Verification items for this drawing (mm, ordinates from the low corner). A direction names the side the tool comes from. Coordinates: 2 decimals unless noted, no trailing zeros. Order: outer loops, then holes, each group sorted by start corner. A loop starts at its lowest first (then second) coordinate and runs counter-clockwise, first axis right, second up. Notation, with made-up numbers: (74, 47) - (85, 47) arc R17 ccw to (85, 79) - close; hole circle Ø7 at (-17, 50). An arc over 180 degrees is marked (long way). Use CSV: the item, a comma, the result in double quotes. Start each with the question number.
1) Sectioned sample at C-C, the plane x = 14. Record the cut outline in (y, z), and give its area (3 significant figures).
2) Sectioned sample at B-B, the plane y = 5.5. Record the cut outline in (x, z).
3) Sectioned sample at A-A, the plane z = 2.25. Record the cut outline in (x, y).
4) Thickness scan on probe 1 along X at (y, z) = (5.5, 4.75); probe 2 along X at (y, z) = (7, 5.5); probe 3 along X at (y, z) = (3.25, 2.25). Record the ranges inside material, lowest first. Write a range as [from, to].
5) Tool access check on the marked faces 4, 5, 6, 7 and 8. Record the directions out of +Z, -Z, +X, -X, +Y, -Y that give a thin tool (end or side, any length) a straight path to the whole face; none if there is none.
6) Draft check along X on the marked faces 1, 2 and 3. Enter one of: released by +X, released by -X, zero draft, split by the parting line, or undercut.
7) Sectioned sample at D-D, the plane y = 10.75. Record the cut outline in (x, z), and give its area (3 significant figures).
8) Depth check by flat-ended pin: P1, Ø1.5, axis at y = 7.5, z = 3.5, coming from the -X side; P2, Ø4, axis at x = 17.5, y = 2, coming from the +Z side; P3, Ø2, axis at x = 31.5, y = 12, coming from the +Z side; P4, Ø1.5, axis at x = 16.5, z = 5.5, coming from the +Y side. Enter the tip coordinate at first touch or a pass-through.
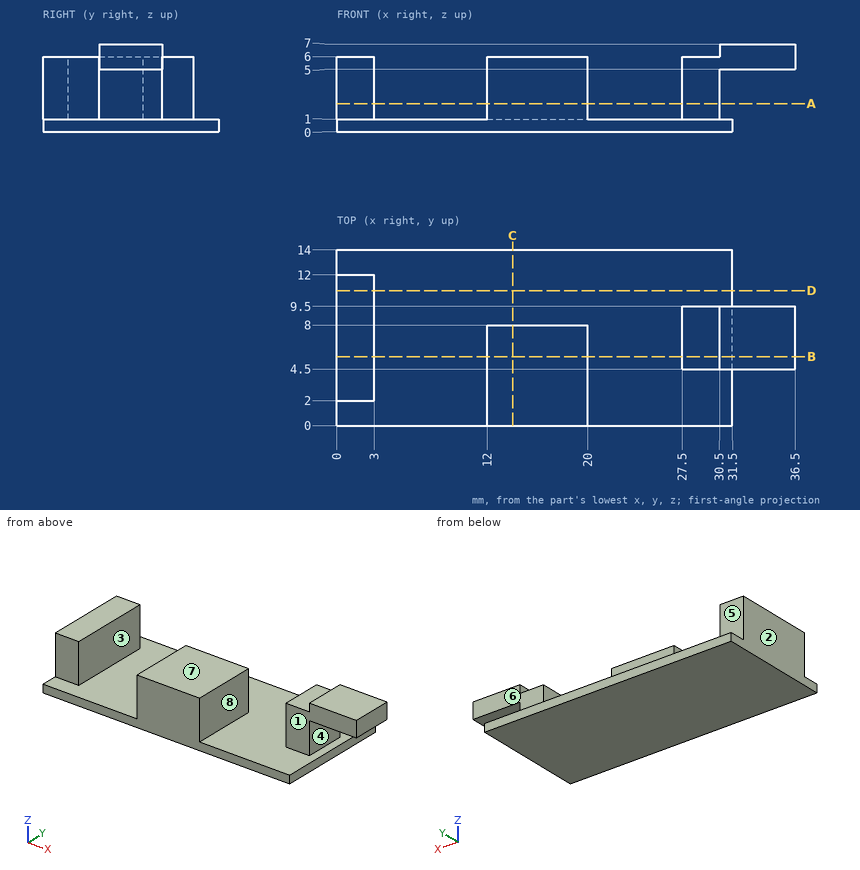
Evaluation:
1,outline,"(0, 0) - (14, 0) - (14, 1) - (8, 1) - (8, 6) - (0, 6) - close"
1,area,"54.0 mm²"
2,outline,"(0, 0) - (31.5, 0) - (31.5, 1) - (30.5, 1) - (30.5, 5) - (36.5, 5) - (36.5, 7) - (30.5, 7) - (30.5, 6) - (27.5, 6) - (27.5, 1) - (20, 1) - (20, 6) - (12, 6) - (12, 1) - (3, 1) - (3, 6) - (0, 6) - close"
3,outline,"(0, 2) - (3, 2) - (3, 12) - (0, 12) - close; (12, 0) - (20, 0) - (20, 8) - (12, 8) - close; (27.5, 4.5) - (30.5, 4.5) - (30.5, 9.5) - (27.5, 9.5) - close"
4,probe 1,"[0, 3], [12, 20], [27.5, 30.5]"
4,probe 2,"[0, 3], [12, 20], [27.5, 36.5]"
4,probe 3,"[0, 3], [12, 20]"
5,face 4,"+X, +Y, -Y"
5,face 5,"+Z, +X, -X, +Y"
5,face 6,"+Z, +X, +Y"
5,face 7,"+Z, -X, +Y, -Y"
5,face 8,"+Z, +Y, -Y"
6,face 1,"zero draft"
6,face 2,"released by -X"
6,face 3,"undercut"
7,outline,"(0, 0) - (31.5, 0) - (31.5, 1) - (3, 1) - (3, 6) - (0, 6) - close"
7,area,"46.5 mm²"
8,P1,"x = 0"
8,P2,"z = 6"
8,P3,"z = 1"
8,P4,"y = 8"
